```python
from build123d import *

# Parameters (mm, degrees)
SHELL1_T            = -3
SKETCH3_R           = 5
BOSS_EXTRUDE1_DEPTH = 30


with BuildPart() as part:
    # Sketch2 → Revolve1 (revolve)
    with BuildSketch(Plane.XY, mode=Mode.PRIVATE) as revolve1_sk:
        with BuildLine():
            Line((0, 0), (0, 53))
            Line((0, 53), (-15, 53))
            ThreePointArc((-15, 53), (-40.721592269, 37.091129978), (-54.166410256, 10))
            Line((-54.166410256, 10), (-49.166410256, 10))
            Line((-49.166410256, 10), (-49.166410256, 0))
            Line((-49.166410256, 0), (0, 0))
        make_face()
    revolve(revolve1_sk.sketch.rotate(Axis((0, 0, 0), (-1, 0, 0)), 90), axis=Axis((0, 0, 0), (-1, 0, 0)))

    # Shell1
    shell1_openings = [part.faces().sort_by_distance(p)[0] for p in [
        (0, 0, 0),
    ]]
    offset(amount=SHELL1_T, openings=shell1_openings, kind=Kind.INTERSECTION)

    # Sketch3 → Boss-Extrude1 (add)
    with BuildSketch(Plane(origin=(-46.166410256, 0, 0), x_dir=(0, 0, -1), z_dir=(1, 0, 0))):
        Circle(SKETCH3_R)
    extrude(amount=BOSS_EXTRUDE1_DEPTH)


solid = part.part
```
The listing builds one solid part. Answer for the finished solid, in the listing's coordinates (mm). A direction names the side the tool comes from. Coordinates: 2 decimals unless noted, no trailing zeros. Loops run counter-clockwise (first coordinate to the right, second up) from the corner with the lowest first, then second, coordinate; pieces in that order, holes last. Notation, with made-up numbers: (-37.5, 89) - (19.5, 89) arc R23 cw to (19.5, 120) - close; hole circle Ø10 at (44.25, 0). An arc over 180 degrees is marked (long way). Write item = value, one per line.
1) Section D-D (z = 30) is taken. Determine the outline of the cut face in (x, y).
Responses:
outline = (-15, -43.69) - (0, -43.69) - (0, -40) - (-14.58, -40) arc R42.57 cw to (-14.58, 40) - (0, 40) - (0, 43.69) - (-15, 43.69) arc R46.2 ccw to start
2) Section C-C (x = -13) is taken. Determine the outline of the cut face in (y, z), plus the area to 3 significant figures.
Responses:
outline = circle Ø106 at (0, 0); hole circle Ø100 at (0, 0)
area = 971 mm^2
3) Find the intervals of material crossed by line 1 along Z through (x, y) = (-28, 2.5); line 2 along Y through (x, z) = (-5, 0); line 3 along Y through (x, z) = (-24, -40.5), in increasing order.
Responses:
line_1 = -47.37 to -43.84, -4.33 to 4.33, 43.84 to 47.37
line_2 = -53 to -50, 50 to 53
line_3 = -28.6 to -22.28, 22.28 to 28.6
4) Which of the six approach directions +Z, -Z, +X, -X, +Y, -Y give full straight-line access (tool end or side, diameter ignored) to faces 4 (the face through (-49.166, 0, 0)), 5 (the face through (-31.38, -4.88, 1.08))?
Responses:
face_4 = -X
face_5 = +X
5) Section A-A (z = 0) is taken. Determine the outline of the cut face in (x, y).
Responses:
outline = (-54.17, -10) arc R55.08 ccw to (-15, -53) - (0, -53) - (0, -50) - (-14.58, -50) arc R52.08 cw to (-50.43, -13) - (-46.17, -13) - (-46.17, -5) - (-16.17, -5) - (-16.17, 5) - (-46.17, 5) - (-46.17, 13) - (-50.43, 13) arc R52.08 cw to (-14.58, 50) - (0, 50) - (0, 53) - (-15, 53) arc R55.08 ccw to (-54.17, 10) - (-49.17, 10) - (-49.17, -10) - close
6) Each of these flat-tipped pins is pushed along its axis until it touches: P1, Ø8, axis at x = -12.5, y = 25, coming from the -Z side; P2, Ø21, axis at y = -6, z = 3, coming from the +X side; P3, Ø5, axis at x = -28.5, y = 9.5, coming from the +Z side. Where does it stop, or does it pass through?
Responses:
P1 = -48.66
P2 = -16.17
P3 = 47.7
7) Determine the mould class of faces 1 (the face through (0, -32, 39)), 2 (the face through (-7.6, -52.55, 6.9)), 3 (the face through (-16.166, 0, 0)) for opening direction Z: pulls with the +Z half, pulls with the -Z half, needs draft (parallel to the pull), parting line crosses it, or undercut.
Responses:
face_1 = needs draft
face_2 = parting line crosses it
face_3 = undercut
